from build123d import *

# Parameters (mm, degrees)
F0_W      = 15.5
F0_H      = 130
F1_DEPTH  = 100
F2_W      = 12
F2_H      = 125
F3_DEPTH  = 95
F4_W      = 20
F4_H      = 5
F4_W_2    = 5.5
F4_H_2    = 5.5
F5_DEPTH  = 1
F6_W      = 2.5
F6_H      = 6.25
F6_R      = 1.75
F7_DEPTH  = 1
F8_W      = 11
F8_H      = 3
F9_DEPTH  = 1
F10_W     = 150
F10_H     = 95
F10_R     = 1.5
F11_DEPTH = 1


with BuildPart() as f1:
    # F0 (on Right) → F1 (new body, symmetric)
    with BuildSketch(Plane.YZ):
        Rectangle(F0_W, F0_H)
    extrude(amount=F1_DEPTH, both=True)


with BuildPart() as f3:
    # F2 (on Right) → F3 (new body, symmetric)
    with BuildSketch(Plane.YZ):
        Rectangle(F2_W, F2_H)
    extrude(amount=F3_DEPTH, both=True)


with BuildPart() as f5_tool:
    # F4 (on face) → F5 (new body)
    with BuildSketch(Plane(origin=(0, 6, 0), x_dir=(-1, 0, 0), z_dir=(0, 1, 0))):
        with Locations((-65, -58)):
            Rectangle(F4_W, F4_H)
        with Locations((65, -58)):
            Rectangle(F4_W, F4_H)
        with Locations((-84.25, 51.75)):
            Rectangle(F4_W_2, F4_H_2)
    extrude(amount=-F5_DEPTH)


with BuildPart() as f1_1:
    add(f1.part)

    # F5: cut by f5_tool
    add(f5_tool.part, mode=Mode.SUBTRACT)


with BuildPart() as f3_1:
    add(f3.part)

    # F5: cut by f5_tool
    add(f5_tool.part, mode=Mode.SUBTRACT)


with BuildPart() as f7_tool:
    # F6 (on face) → F7 (new body)
    with BuildSketch(Plane.YZ.offset(95)):
        with Locations((0, -30.625)):
            Rectangle(F6_W, F6_H)
        with Locations((0, -41.375)):
            Rectangle(F6_W, F6_H)
        with Locations((0, 41.5)):
            Circle(F6_R)
    extrude(amount=-F7_DEPTH)


with BuildPart() as f1_2:
    add(f1_1.part)

    # F7: cut by f7_tool
    add(f7_tool.part, mode=Mode.SUBTRACT)


with BuildPart() as f3_2:
    add(f3_1.part)

    # F7: cut by f7_tool
    add(f7_tool.part, mode=Mode.SUBTRACT)


with BuildPart() as f9_tool:
    # F8 (on face) → F9 (new body)
    with BuildSketch(Plane.XY.offset(62.5)):
        with Locations((57.5, 0)):
            Rectangle(F8_W, F8_H)
        with Locations((69.5, 0)):
            Rectangle(F8_W, F8_H)
    extrude(amount=-F9_DEPTH)


with BuildPart() as f1_3:
    add(f1_2.part)

    # F9: cut by f9_tool
    add(f9_tool.part, mode=Mode.SUBTRACT)


with BuildPart() as f3_3:
    add(f3_2.part)

    # F9: cut by f9_tool
    add(f9_tool.part, mode=Mode.SUBTRACT)


with BuildPart() as f11_tool:
    # F10 (on face) → F11 (new body)
    with BuildSketch(Plane.XZ.offset(6)):
        Rectangle(F10_W, F10_H)
        with Locations((84, 0)):
            Circle(F10_R)
    extrude(amount=-F11_DEPTH)


with BuildPart() as f1_4:
    add(f1_3.part)

    # F11: cut by f11_tool
    add(f11_tool.part, mode=Mode.SUBTRACT)


with BuildPart() as f3_4:
    add(f3_3.part)

    # F11: cut by f11_tool
    add(f11_tool.part, mode=Mode.SUBTRACT)


solid = f3_4.part
Can you work these out from the model? Positions are in its coordinate system, mm. A direction names the side the tool comes from. Round coordinates to 2 decimals unless told otherwise and drop trailing zeros. Order: outer loops, then holes, each group sorted by start corner. A loop starts at its lowest first (then second) coordinate and runs counter-clockwise, first axis right, second up. Notation, with made-up numbers: (20.5, -2.75) -> (71.5, -2.75) arc R24 ccw to (71.5, 24.25) -> close; hole circle Ø8 at (14.25, 22). An arc over 180 degrees is marked (long way). Write each question's results on one line, items separated by ' | '. Start each with the question number.
Item 1: If we section it at B-B, the plane x = -13: Write out the boundary of the cut face in (y, z), then the cut area to 4 significant figures.
Item 2: Will these pins go through, and if not, where does the flat tip stop? pin 1 (1 mm diameter, centred on y = 0.5, z = 41.5, fed in from +X); pin 2 (1.6 mm diameter, centred on x = 83.5, z = 53, fed in from +Y).
Item 3: Thinking about a two-plate mould opening in Z: for faces 1 (the flat face through (1, 0, -62.5)), 2 (the flat face through (-1, -5, 1)), 3 (the flat face through (-95, 0, 1)), which applies, +Z half, -Z half, draft (parallel to the pull), parting line (faces both ways), or undercut?
Item 4: Please list where these lines run through material, in increasing order: L1, parallel to Z at x = 94.8, y = 0; L2, parallel to Z at x = 84, y = -5.25; L3, parallel to Y at x = -31.5, z = 9.
Item 5: Which directions (+Z, -Z, +X, -X, +Y, -Y) give clear straight access to the entire face, cutting with the end or side of a thin tool? Please do faces 4 (the flat face through (-65, 5, -58)), 5 (the cylindrical face through (94.51, -0.38, 39.79)), 6 (the flat face through (1, 0, 62.5)).
Item 6: If we section it at A-A, the plane z = -19: Write out the boundary of the cut face in (x, y), then the cut area to 3 significant figures.
Results:
1) outline: (-6, -62.5) -> (6, -62.5) -> (6, 62.5) -> (-6, 62.5) -> (-6, 47.5) -> (-5, 47.5) -> (-5, -47.5) -> (-6, -47.5) -> close | area: 1,405 mm2
2) pin 1: stops at x = 94 | pin 2: stops at y = 5
3) face 1: -Z half | face 2: undercut | face 3: draft
4) L1: z = -62.5 to -44.5, -38.25 to -33.75, -27.5 to 39.75, 43.25 to 62.5 | L2: z = -62.5 to -1.5, 1.5 to 62.5 | L3: y = -5 to 6
5) face 4: +Y | face 5: +X | face 6: +Z, +X, -X, +Y, -Y
6) outline: (-95, -6) -> (-75, -6) -> (-75, -5) -> (75, -5) -> (75, -6) -> (95, -6) -> (95, 6) -> (-95, 6) -> close | area: 2,130 mm2
